Can you work these out from the drawing? Everything is in mm from the part's minimum corner. A direction names the side the tool comes from. Coordinates: 2 decimals unless noted, no trailing zeros. Order: outer loops, then holes, each group sorted by start corner. A loop starts at its lowest first (then second) coordinate and runs counter-clockwise, first axis right, second up. Notation, with made-up numbers: (11, 88) -> (50, 88) arc R22 ccw to (50, 105) -> close; hole circle Ø6 at (39, -34). An arc over 180 degrees is marked (long way). Answer in a Markdown table with one row per item.
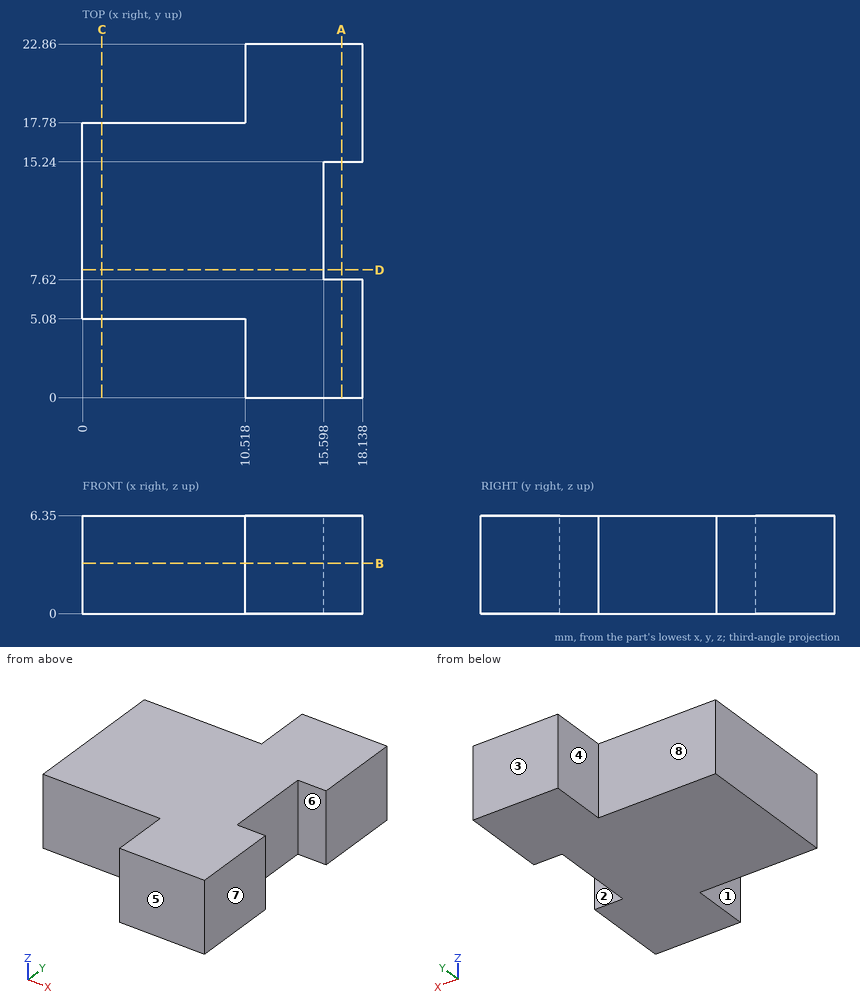
(1) On a 3-axis mill with a long thin cutter (end or side, diameter ignored), from which of +Z, -Z, +X, -X, +Y, -Y can I reach the whole of each face in a straight line? I mean the marked faces 1, 2, 3, 4 and 5. Say none if no direction works.
Response values:
| item | result |
|---|---|
| face 1 | +Z, -Z, -X, -Y |
| face 2 | +Z, -Z, +X |
| face 3 | +Z, -Z, +X, -X, +Y |
| face 4 | +Z, -Z, -X, +Y |
| face 5 | +Z, -Z, +X, -X, -Y |
(2) We'd pull the mould along Y, two halves only. Please class the marked faces 6, 7 and 8: +Y half, -Y half, draft (parallel to the pull), parting line (faces both ways), or undercut.
Response values:
| item | result |
|---|---|
| face 6 | undercut |
| face 7 | draft |
| face 8 | +Y half |
(3) Suppose I cut it at A-A (x = 16.75). Please give me the cut outline in (y, z).
Response values:
| item | result |
|---|---|
| outline | (0, 0) -> (7.62, 0) -> (7.62, 6.35) -> (0, 6.35) -> close; (15.24, 0) -> (22.86, 0) -> (22.86, 6.35) -> (15.24, 6.35) -> close |
(4) I need wall thicknesses on line 1 (Y direction, x = 17.75, z = 5.5); line 2 (Y direction, x = 2.25, z = 1.5); line 3 (X direction, y = 3.5, z = 5.5). Which ranges of each line are inside material? Lowest first, please. Write a range as [from, to].
Response values:
| item | result |
|---|---|
| line 1 | [0, 7.62], [15.24, 22.86] |
| line 2 | [5.08, 17.78] |
| line 3 | [10.52, 18.14] |
(5) Suppose I cut it at D-D (y = 8.25). Please give me the cut outline in (x, z).
Response values:
| item | result |
|---|---|
| outline | (0, 0) -> (15.6, 0) -> (15.6, 6.35) -> (0, 6.35) -> close |
(6) Suppose I cut it at C-C (x = 1.25). Please give me the cut outline in (y, z).
Response values:
| item | result |
|---|---|
| outline | (5.08, 0) -> (17.78, 0) -> (17.78, 6.35) -> (5.08, 6.35) -> close |
(7) Will these pins go through, and if not, where does the flat tip stop? pin 1 Ø8 at (x, y) = (7, 19) entering from -Z; pin 2 Ø1.9 at (x, z) = (7, 2) entering from +Y; pin 3 Ø1.5 at (y, z) = (19.5, 2) entering from -X; pin 4 Ø3 at (y, z) = (9.5, 4.5) entering from +X.
Response values:
| item | result |
|---|---|
| pin 1 | z = 0 |
| pin 2 | y = 17.78 |
| pin 3 | x = 10.52 |
| pin 4 | x = 15.6 |
(8) Suppose I cut it at B-B (z = 3.25). Please give me the cut outline in (x, y).
Response values:
| item | result |
|---|---|
| outline | (0, 5.08) -> (10.52, 5.08) -> (10.52, 0) -> (18.14, 0) -> (18.14, 7.62) -> (15.6, 7.62) -> (15.6, 15.24) -> (18.14, 15.24) -> (18.14, 22.86) -> (10.52, 22.86) -> (10.52, 17.78) -> (0, 17.78) -> close |
